```python
from build123d import *

# Parameters (mm, degrees)
SKETCH1_W           = 29
SKETCH1_H           = 29
BOSS_EXTRUDE1_DEPTH = 2
SKETCH2_W           = 12
SKETCH2_H           = 12
BOSS_EXTRUDE2_DEPTH = 3
SKETCH5_R           = 5
BOSS_EXTRUDE3_DEPTH = 5
SKETCH6_R           = 4
BOSS_EXTRUDE4_DEPTH = 2
SKETCH8_R           = 6
SKETCH8_R_2         = 5
EXTRUDE_THIN2_DEPTH = 6
SKETCH9_R           = 5
BOSS_EXTRUDE5_DEPTH = 0.5
REVOLVE1_ANGLE      = 180


with BuildPart() as part:
    # Sketch1 → Boss-Extrude1 (new body)
    with BuildSketch(Plane(origin=(0, 0, 0), x_dir=(1, 0, 0), z_dir=(0, 1, 0))):
        with Locations((14.5, 14.5)):
            Rectangle(SKETCH1_W, SKETCH1_H)
    extrude(amount=BOSS_EXTRUDE1_DEPTH)

    # Sketch2 → Boss-Extrude2 (add)
    with BuildSketch(Plane(origin=(0, 2, 0), x_dir=(1, 0, 0), z_dir=(0, 1, 0))):
        with Locations((14.566374873, 14.72560783)):
            Rectangle(SKETCH2_W, SKETCH2_H)
    extrude(amount=BOSS_EXTRUDE2_DEPTH)

    # Sketch5 → Boss-Extrude3 (add)
    with BuildSketch(Plane(origin=(0, 5, 0), x_dir=(1, 0, 0), z_dir=(0, 1, 0))):
        with Locations(Location((14.566374873, 14.72560783, 0), (0, 0, 270))):
            Circle(SKETCH5_R)
    extrude(amount=BOSS_EXTRUDE3_DEPTH)

    # Sketch6 → Boss-Extrude4 (add)
    with BuildSketch(Plane(origin=(0, 10, 0), x_dir=(1, 0, 0), z_dir=(0, 1, 0))):
        with Locations(Location((14.566374873, 14.72560783, 0), (0, 0, 270))):
            Circle(SKETCH6_R)
    extrude(amount=BOSS_EXTRUDE4_DEPTH)



with BuildPart() as body_2:
    # Sketch8 → Extrude-Thin2 (new body)
    with BuildSketch(Plane(origin=(0, 12, 0), x_dir=(1, 0, 0), z_dir=(0, 1, 0))):
        with Locations((14.566374873, 14.72560783)):
            Circle(SKETCH8_R)
        with Locations((14.566374873, 14.72560783)):
            Circle(SKETCH8_R_2, mode=Mode.SUBTRACT)
    extrude(amount=EXTRUDE_THIN2_DEPTH)


with BuildPart() as part_1:
    add(part.part)

    add(body_2.part)  # Boss-Extrude5 merges body 2
    # Sketch9 → Boss-Extrude5 (add)
    with BuildSketch(Plane(origin=(0, 12, 0), x_dir=(1, 0, 0), z_dir=(0, 1, 0))):
        with Locations(Location((14.566374873, 14.72560783, 0), (0, 0, 270))):
            Circle(SKETCH9_R)
    extrude(amount=BOSS_EXTRUDE5_DEPTH)

    # Sketch13 → Revolve1 (revolve)
    with BuildSketch(Plane(origin=(0, 12.5, 0), x_dir=(1, 0, 0), z_dir=(0, 1, 0))):
        with BuildLine():
            Line((9.847526331, 16.378625808), (19.285223415, 13.072589852))
            ThreePointArc((19.285223415, 13.072589852), (16.219392851, 19.444456372), (9.847526331, 16.378625808))
        make_face()
    revolve(axis=Axis((9.847526331, 12.5, -16.378625808), (0.9437697084535585, 0, 0.33060359557253066)), revolution_arc=REVOLVE1_ANGLE)


solid = part_1.part
```
Input: part model. Units: mm. Frame: model coordinates. A direction names the side the tool comes from. Give positions to 0.01 mm unless a question says otherwise; leave off trailing zeros. Write each loop counter-clockwise with the first axis right and the second up, starting at its lowest first coordinate (ties: lowest second). Pieces come first, ordered by that corner, then holes. Notation, with made-up numbers: (8, -0.5) - (35, -0.5) arc R16 ccw to (35, 9.5) - close; hole circle Ø9 at (28, 56.25). An arc over 180 degrees is marked (long way). Write item = value, one per line. Start each with the question number.
1. Mould query, pull axis Y, two halves, no side actions, for faces 6 (the flat face through (19, 10, -15)), 7 (the flat face through (14, 0, -15)), 8 (the flat face through (0, 1, -14)). Classes: released by +Y, released by -Y, zero draft, split by the parting line, or undercut.
2. Section query B-B, the plane y = 13.5. Output: boundary loops of the cut face in (x, z), then the cut area to 3 significant figures.
3. Section query C-C, the plane x = 17.75. Output: boundary loops of the cut face in (y, z).
4. Section query D-D, the plane y = 3.75. Output: boundary loops of the cut face in (x, z).
5. Ray query, L1, parallel to Z at x = 12.25, y = 15.25; L2, parallel to X at y = 14.5, z = -13.25; L3, parallel to Z at x = 10.75, y = 14. Return the intervals inside material, ascending.
6. Section query A-A, the plane z = -12. Output: boundary loops of the cut face in (x, y), then the cut area to 3 significant figures.
7. First-contact query: pin 1 Ø1.5 at (x, z) = (3.5, -24.5) entering from +Y; pin 2 Ø1.5 at (y, z) = (8, -17) entering from +X; pin 3 Ø0.9 at (x, y) = (13, 3.5) entering from -Z. Flat tips, straight axial feed; report the tip coordinate or a pass-through.
8. Access query for faces 1 (the flat face through (14, 3, -20.726)), 2 (the flat face through (20.566, 3, -15)), 3 (the cylindrical face through (20.3, 15, -16.5)), 4 (the cylindrical face through (11.018, 10.986, -12.88)), 5 (the flat face through (14, 3, -8.726)). Directions: +Z, -Z, +X, -X, +Y, -Y. A direction counts if a zero-diameter tool reaches every point of the face in a straight line with its end or side. Return the directions, or none.
Check sheet entries:
q1.face_6 = undercut
q1.face_7 = released by -Y
q1.face_8 = zero draft
q2.outline = circle Ø12 at (14.57, -14.73); circle Ø9.8 at (14.57, -14.73); hole circle Ø10 at (14.57, -14.73)
q2.area = 110 mm2
q3.outline = (0, -29) - (2, -29) - (2, -20.73) - (5, -20.73) - (5, -18.58) - (10, -18.58) - (10, -17.15) - (12, -17.15) - (12, -19.81) - (18, -19.81) - (18, -18.58) - (12.5, -18.58) arc R3.86 ccw to (12.5, -10.87) - (18, -10.87) - (18, -9.64) - (12, -9.64) - (12, -12.3) - (10, -12.3) - (10, -10.87) - (5, -10.87) - (5, -8.73) - (2, -8.73) - (2, 0) - (0, 0) - close
q4.outline = (8.57, -20.73) - (20.57, -20.73) - (20.57, -8.73) - (8.57, -8.73) - close
q5.L1 = -20.26 to -19.16, -18.2 to -11.25, -10.29 to -9.19
q5.L2 = 8.75 to 9.79, 10.23 to 18.9, 19.34 to 20.38
q5.L3 = -19.36 to -17.96, -17.59 to -11.86, -11.5 to -10.1
q6.outline = (0, 0) - (29, 0) - (29, 2) - (20.57, 2) - (20.57, 5) - (18.76, 5) - (18.76, 10) - (17.49, 10) - (17.49, 12) - (19.91, 12) - (19.91, 18) - (18.76, 18) - (18.76, 12.5) arc R4.19 ccw to (10.37, 12.5) - (10.37, 18) - (9.22, 18) - (9.22, 12) - (11.64, 12) - (11.64, 10) - (10.37, 10) - (10.37, 5) - (8.57, 5) - (8.57, 2) - (0, 2) - close
q6.area = 193 mm2
q7.pin_1 = 2
q7.pin_2 = 19.33
q7.pin_3 = -20.73
q8.face_1 = -Z, +X, -X, +Y
q8.face_2 = +Z, -Z, +X, +Y
q8.face_3 = +Y
q8.face_4 = none
q8.face_5 = +Z, +X, -X, +Y
